from build123d import *

# Parameters (mm, degrees)
SKETCH1_W           = 82
SKETCH1_H           = 82
BOSS_EXTRUDE1_DEPTH = 12
SKETCH2_R           = 1.5
CUT_EXTRUDE1_DEPTH  = 106.677700072
SKETCH3_R           = 41
BOSS_EXTRUDE2_DEPTH = 15
SKETCH4_R           = 1.5
CUT_EXTRUDE2_DEPTH  = 5


with BuildPart() as part:
    # Sketch1 → Boss-Extrude1 (new body)
    with BuildSketch(Plane(origin=(0, 0, 0), x_dir=(1, 0, 0), z_dir=(0, 1, 0))):
        with Locations((-48.046875, -14.627604167)):
            Rectangle(SKETCH1_W, SKETCH1_H)
    extrude(amount=BOSS_EXTRUDE1_DEPTH)

    # Sketch2 → Cut-Extrude1 (cut, through all)
    with BuildSketch(Plane.XZ):
        with Locations(Location((-85.546875, 52.127604167, 0), (0, 0, 270))):
            Circle(SKETCH2_R)
        with Locations(Location((-10.546875, 52.127604167, 0), (0, 0, 270))):
            Circle(SKETCH2_R)
        with Locations(Location((-85.546875, -22.872395833, 0), (0, 0, 270))):
            Circle(SKETCH2_R)
        with Locations(Location((-10.546875, -22.872395833, 0), (0, 0, 270))):
            Circle(SKETCH2_R)
    extrude(amount=-CUT_EXTRUDE1_DEPTH, mode=Mode.SUBTRACT)

    # Sketch3 → Boss-Extrude2 (add)
    with BuildSketch(Plane(origin=(0, 12, 0), x_dir=(1, 0, 0), z_dir=(0, 1, 0))):
        with Locations(Location((-48.046875, -14.627604167, 0), (0, 0, 270))):
            Circle(SKETCH3_R)
    extrude(amount=BOSS_EXTRUDE2_DEPTH)

    # Sketch4 → Cut-Extrude2 (cut)
    with BuildSketch(Plane.XZ):
        with Locations(Location((-57.046875, 14.877604167, 0), (0, 0, 270))):
            Circle(SKETCH4_R)
        with Locations(Location((-39.046875, 14.877604167, 0), (0, 0, 270))):
            Circle(SKETCH4_R)
    extrude(amount=-CUT_EXTRUDE2_DEPTH, mode=Mode.SUBTRACT)


solid = part.part
Design review of the part built by this model. Coordinates are the model's own, in mm. A direction names the side the tool comes from. Coordinates: 2 decimals unless noted, no trailing zeros. Order: outer loops, then holes, each group sorted by start corner. A loop starts at its lowest first (then second) coordinate and runs counter-clockwise, first axis right, second up. Notation, with made-up numbers: (87.25, -9) -> (126.25, -9) arc R25 ccw to (126.25, 22) -> close; hole circle Ø7 at (59, 60.25). An arc over 180 degrees is marked (long way). One line per item, written item: value.
1) We need section A-A, the plane z = 37. Give the boundary of the cut face in (x, y).
Output values:
outline: (-89.05, 0) -> (-7.05, 0) -> (-7.05, 12) -> (-13.69, 12) -> (-13.69, 27) -> (-82.4, 27) -> (-82.4, 12) -> (-89.05, 12) -> close
2) Draft analysis for pull direction X (two halves, no side actions). For faces 4 (the face through (-40.38, 2.46, 14.19)), 5 (the face through (-79, 12, 47)), 6 (the face through (-84.282, 5.916, 51.321)), 7 (the face through (-88.07, 19.4, 5.74)), state which applies: +X half, -X half, draft (parallel to the pull), parting line (faces both ways), or undercut.
Output values:
face 4: undercut
face 5: draft
face 6: undercut
face 7: parting line
3) We need section C-C, the plane y = 15. Give the boundary of the cut face in (x, z).
Output values:
outline: circle Ø82 at (-48.05, 14.63)
4) Clearance check with flat-ended pins moving along their axes: P1, Ø5, axis at x = -85.55, z = 52.13, coming from the +Y side; P2, Ø2, axis at x = -37.5, y = 16.5, coming from the -Z side; P3, Ø8, axis at y = 18.5, z = 33.5, coming from the +X side. State where each tip first meets the part, or that it passes through.
Output values:
P1: stops at y = 12
P2: stops at z = -25.25
P3: stops at x = -9.84
5) Machinability: for faces 1 (the face through (-15, 12, 47)), 2 (the face through (-79, 12, -17)), 3 (the face through (-39, 5, 15)), which of the approach directions +Z, -Z, +X, -X, +Y, -Y give a long, thin tool a straight path to every point of the face, cutting with its end or side? Answer none if there is none.
Output values:
face 1: +Z, +X, +Y
face 2: -Z, -X, +Y
face 3: -Y
6) We need section B-B, the plane x = -82. Give the boundary of the cut face in (y, z), then the cut area to 3 significant figures.
Output values:
outline: (0, -26.37) -> (12, -26.37) -> (12, -8.35) -> (27, -8.35) -> (27, 37.61) -> (12, 37.61) -> (12, 55.63) -> (0, 55.63) -> close
area: 1,670 mm2
7) To check wall thickness, follow probe 1 along Z at (x, y) = (-11.5, 8.75); probe 2 along Y at (x, z) = (-74.5, 52.5); probe 3 along X at (y, z) = (20, 2). State the ranges of each line that lie inside material, in increasing order. Write a range as [from, to].
Output values:
probe 1: z = [-26.37, -24.03], [-21.71, 50.97], [53.29, 55.63]
probe 2: y = [0, 12]
probe 3: x = [-87.05, -9.04]
